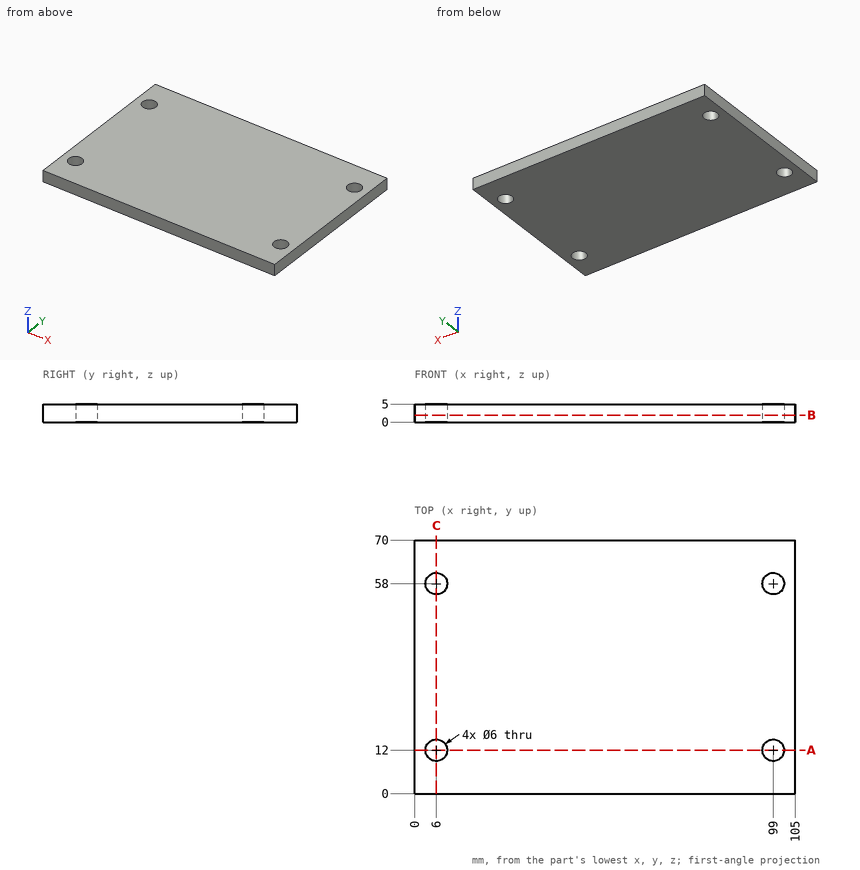
Part print with two shaded views. Sizes in mm from the minimum x, y, z corner. Coordinates: 2 decimals unless noted, no trailing zeros. Order: outer loops, then holes, each group sorted by start corner. A loop starts at its lowest first (then second) coordinate and runs counter-clockwise, first axis right, second up. Notation, with made-up numbers: (-32, 18) - (1, 18) arc R15 ccw to (1, 34) - close; hole circle Ø1 at (20.25, -13.5). An arc over 180 degrees is marked (long way). Answer in a Markdown table with one row per item.
1. Flat gauge pin, fed straight in: P1, Ø8, axis at x = 99, y = 12, coming from the -Z side. Where does the tip first touch, or does it go through?
Answer:
| item | result |
|---|---|
| P1 | z = 0 |
2. Slice it at C-C, the plane x = 6. List the corners of the cut face in (y, z), then the cut area to 3 significant figures.
Answer:
| item | result |
|---|---|
| outline | (0, 0) - (9, 0) - (9, 5) - (0, 5) - close; (15, 0) - (55, 0) - (55, 5) - (15, 5) - close; (61, 0) - (70, 0) - (70, 5) - (61, 5) - close |
| area | 290 mm² |
3. Slice it at B-B, the plane z = 1.95. List the corners of the cut face in (x, y), then the cut area to 3 significant figures.
Answer:
| item | result |
|---|---|
| outline | (0, 0) - (105, 0) - (105, 70) - (0, 70) - close; hole circle Ø6 at (6, 12); hole circle Ø6 at (6, 58); hole circle Ø6 at (99, 12); hole circle Ø6 at (99, 58) |
| area | 7,240 mm² |
4. Drill centre lines: L1, parallel to Y at x = 6, z = 3.9; L2, parallel to X at y = 55.5, z = 2.45; L3, parallel to X at y = 13.5, z = 3.95. Where is each one in solid material? Low to high. Write a range as from..to.
Answer:
| item | result |
|---|---|
| L1 | 0..9, 15..55, 61..70 |
| L2 | 0..4.34, 7.66..97.34, 100.66..105 |
| L3 | 0..3.4, 8.6..96.4, 101.6..105 |
5. Slice it at A-A, the plane y = 12. List the corners of the cut face in (x, z), then the cut area to 3 significant figures.
Answer:
| item | result |
|---|---|
| outline | (0, 0) - (3, 0) - (3, 5) - (0, 5) - close; (9, 0) - (96, 0) - (96, 5) - (9, 5) - close; (102, 0) - (105, 0) - (105, 5) - (102, 5) - close |
| area | 465 mm² |
